Could you check a few things on this drawing? It's one solid part, dimensions in mm from its lowest x, y, z. Coordinates: 2 decimals unless noted, no trailing zeros. Order: outer loops, then holes, each group sorted by start corner. A loop starts at its lowest first (then second) coordinate and runs counter-clockwise, first axis right, second up. Notation, with made-up numbers: (8.5, 59) - (38.5, 59) arc R33 ccw to (38.5, 90) - close; hole circle Ø2 at (89, 29.5). An arc over 180 degrees is marked (long way). Return JSON: item names as keys, results as strings. Group by question number.
1) For pin 1 Ø0.9 at (x, z) = (48, 1.5) entering from -Y, with a flat end and sliding along its axis, tell me the tip position at first contact or that it passes through.
2) Imagine slicing it at A-A (z = 13). Write out the boundary of the cut face in (x, y).
3) Imagine slicing it at B-B (x = 124.2). Write out the boundary of the cut face in (y, z).
4) If I drill on line 1 along Y through (x, z) = (9.8, 10); line 2 along Y through (x, z) = (124.2, 3.5), over which ranges is the centre line in solid material (lowest first)?
5) Imagine slicing it at D-D (x = 33.5). Write out the boundary of the cut face in (y, z).
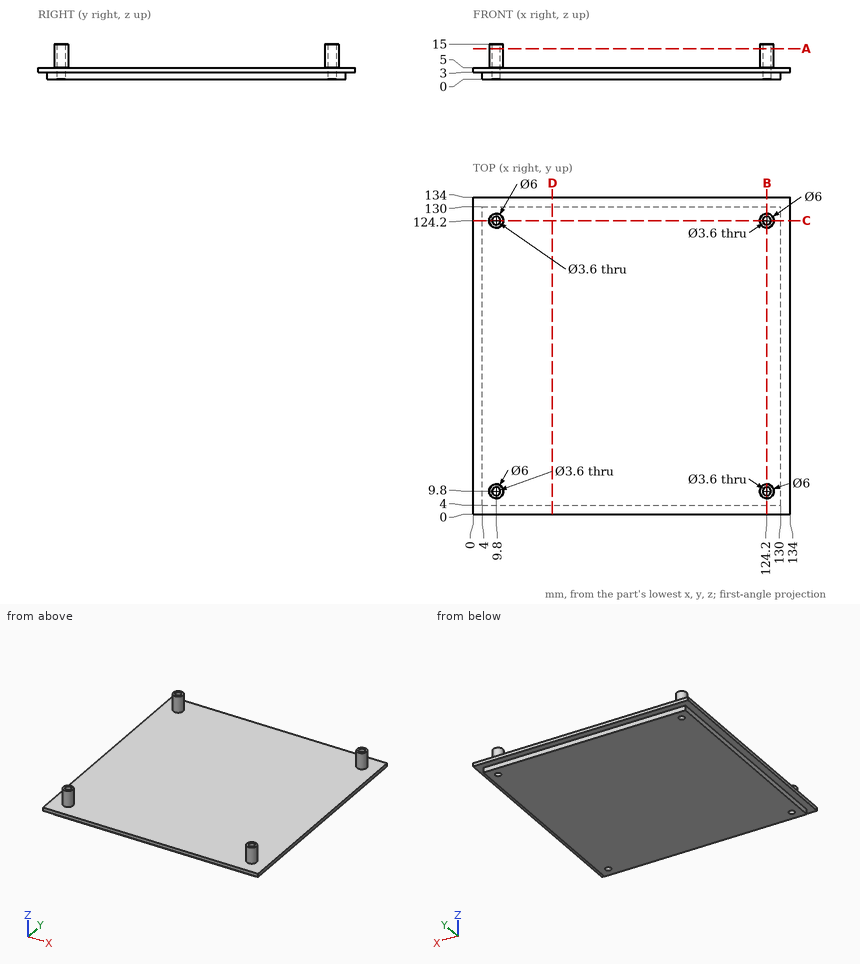
Calculated:
{
 "1": {"pin 1": "y = 4"},
 "2": {"outline": "circle Ø6 at (9.8, 9.8); circle Ø6 at (9.8, 124.2); circle Ø6 at (124.2, 9.8); circle Ø6 at (124.2, 124.2); hole circle Ø3.6 at (9.8, 9.8); hole circle Ø3.6 at (9.8, 124.2); hole circle Ø3.6 at (124.2, 9.8); hole circle Ø3.6 at (124.2, 124.2)"},
 "3": {"outline": "(0, 3) - (4, 3) - (4, 0) - (8, 0) - (8, 15) - (6.8, 15) - (6.8, 5) - (0, 5) - close; (11.6, 0) - (122.4, 0) - (122.4, 15) - (121.2, 15) - (121.2, 5) - (12.8, 5) - (12.8, 15) - (11.6, 15) - close; (126, 0) - (130, 0) - (130, 3) - (134, 3) - (134, 5) - (127.2, 5) - (127.2, 15) - (126, 15) - close"},
 "4": {"line 1": "6.8 to 8, 11.6 to 12.8, 121.2 to 122.4, 126 to 127.2", "line 2": "0 to 8, 11.6 to 122.4, 126 to 134"},
 "5": {"outline": "(0, 3) - (4, 3) - (4, 0) - (130, 0) - (130, 3) - (134, 3) - (134, 5) - (0, 5) - close"}
}
